```python
from build123d import *

# Parameters (mm, degrees)
F0_R     = 5
F1_DEPTH = 7
F2_DEPTH = 9
F3_R     = 5
F3_R_2   = 3
F4_DEPTH = 4
F5_DEPTH = 14
F6_R     = 1.5
F7_DEPTH = 12.5


with BuildPart() as f1:
    # F0 (on Top) → F1 (new body)
    with BuildSketch(Plane.XY):
        Circle(F0_R)
        with BuildLine():
            ThreePointArc((-2, 1.5), (0, 2.5), (2, 1.5))
            Line((2, 1.5), (3.6073317751, 1.5))
            Line((3.6073317751, 1.5), (3.6073317751, -1.5))
            Line((3.6073317751, -1.5), (2, -1.5))
            ThreePointArc((2, -1.5), (0, -2.5), (-2, -1.5))
            Line((-2, -1.5), (-3.6073317751, -1.5))
            Line((-3.6073317751, -1.5), (-3.6073317751, 1.5))
            Line((-3.6073317751, 1.5), (-2, 1.5))
        make_face(mode=Mode.SUBTRACT)
        with BuildLine():
            ThreePointArc((2, 1.5), (2.3717082451, 0.790569415), (2.5, 0))
            ThreePointArc((2.5, 0), (2.3717082451, -0.790569415), (2, -1.5))
            Line((2, -1.5), (3.6073317751, -1.5))
            Line((3.6073317751, -1.5), (3.6073317751, 1.5))
            Line((3.6073317751, 1.5), (2, 1.5))
        make_face()
        with BuildLine():
            Line((-2, 1.5), (2, 1.5))
            ThreePointArc((2, 1.5), (0, 2.5), (-2, 1.5))
        make_face()
        with BuildLine():
            ThreePointArc((-2, -1.5), (0, -2.5), (2, -1.5))
            Line((2, -1.5), (-2, -1.5))
        make_face()
        with BuildLine():
            ThreePointArc((-2, -1.5), (-2.5, 0), (-2, 1.5))
            Line((-2, 1.5), (-3.6073317751, 1.5))
            Line((-3.6073317751, 1.5), (-3.6073317751, -1.5))
            Line((-3.6073317751, -1.5), (-2, -1.5))
        make_face()
    extrude(amount=F1_DEPTH)

    # F0 (on Top) → F2 (join)
    with BuildSketch(Plane.XY):
        Circle(F0_R)
        with BuildLine():
            ThreePointArc((-2, 1.5), (0, 2.5), (2, 1.5))
            Line((2, 1.5), (3.6073317751, 1.5))
            Line((3.6073317751, 1.5), (3.6073317751, -1.5))
            Line((3.6073317751, -1.5), (2, -1.5))
            ThreePointArc((2, -1.5), (0, -2.5), (-2, -1.5))
            Line((-2, -1.5), (-3.6073317751, -1.5))
            Line((-3.6073317751, -1.5), (-3.6073317751, 1.5))
            Line((-3.6073317751, 1.5), (-2, 1.5))
        make_face(mode=Mode.SUBTRACT)
        with BuildLine():
            ThreePointArc((-2, -1.5), (-2.5, 0), (-2, 1.5))
            Line((-2, 1.5), (-3.6073317751, 1.5))
            Line((-3.6073317751, 1.5), (-3.6073317751, -1.5))
            Line((-3.6073317751, -1.5), (-2, -1.5))
        make_face()
        with BuildLine():
            ThreePointArc((2, 1.5), (2.3717082451, 0.790569415), (2.5, 0))
            ThreePointArc((2.5, 0), (2.3717082451, -0.790569415), (2, -1.5))
            Line((2, -1.5), (3.6073317751, -1.5))
            Line((3.6073317751, -1.5), (3.6073317751, 1.5))
            Line((3.6073317751, 1.5), (2, 1.5))
        make_face()
    extrude(amount=F2_DEPTH)

    # F3 (on face) → F4 (join)
    with BuildSketch(Plane(origin=(0, 0, 0), x_dir=(1, 0, 0), z_dir=(0, 0, -1))):
        Circle(F3_R)
        Circle(F3_R_2, mode=Mode.SUBTRACT)
        Circle(F3_R_2)
        with BuildLine():
            Line((2, -1.5), (-2, -1.5))
            ThreePointArc((-2, -1.5), (-2.5, 0), (-2, 1.5))
            Line((-2, 1.5), (2, 1.5))
            ThreePointArc((2, 1.5), (2.5, 0), (2, -1.5))
        make_face(mode=Mode.SUBTRACT)
        with BuildLine():
            ThreePointArc((-2, 1.5), (-2.5, 0), (-2, -1.5))
            Line((-2, -1.5), (2, -1.5))
            ThreePointArc((2, -1.5), (2.5, 0), (2, 1.5))
            Line((2, 1.5), (-2, 1.5))
        make_face()
    extrude(amount=F4_DEPTH)

    # F3 (on face) → F5 (join)
    with BuildSketch(Plane(origin=(0, 0, 0), x_dir=(1, 0, 0), z_dir=(0, 0, -1))):
        Circle(F3_R)
        Circle(F3_R_2, mode=Mode.SUBTRACT)
    extrude(amount=F5_DEPTH)

    # F6 (on Right) → F7 (cut, symmetric)
    with BuildSketch(Plane.YZ):
        with Locations((0, -5.9965602363)):
            Circle(F6_R)
    extrude(amount=F7_DEPTH, both=True, mode=Mode.SUBTRACT)


solid = f1.part
```
Geometry check sheet. Reference: the model listing, model coordinates, mm. A direction names the side the tool comes from. Give positions to 0.01 mm unless a question says otherwise; leave off trailing zeros. Order: outer loops, then holes, each group sorted by start corner. A loop starts at its lowest first (then second) coordinate and runs counter-clockwise, first axis right, second up.
1. Gauge pin test, flat ends, axial feed: pin 1 Ø1 at (x, z) = (3.5, -8.5) entering from -Y; pin 2 Ø1 at (x, y) = (-1, 2) entering from -Z; pin 3 Ø2.5 at (y, z) = (0, -6) entering from +X; pin 4 Ø1.5 at (x, y) = (0, 0.5) entering from +Z. Record the tip position at first contact, or that the pin passes through.
2. Thickness scan on L1, parallel to X at y = 0, z = -7.75; L2, parallel to Z at x = 1, y = -1.75. Record the ranges inside material, lowest first.
3. Section check C-C, the plane x = 0. Enter the section's corners in (y, z).
4. Section check B-B, the plane z = -6.25. Enter the section's corners in (x, y).
5. Section check A-A, the plane y = 0. Enter the section's corners in (x, z).
6. Access from +Z, -Z, +X, -X, +Y, -Y to the whole of each face (thin tool, end or side, straight path). Record for faces 1 (the face through (0, 1.5, 3)), 2 (the face through (2, -2, 9)).
7. Release check for a two-part mould opening along Y. For faces 3 (the face through (0, 0, -4)), 4 (the face through (-3, 0, -9)), 5 (the face through (-0.1, 3.3, -14)), 6 (the face through (4.77, -1.5, -2.34)) record: pulls with the +Y half, pulls with the -Y half, needs draft (parallel to the pull), parting line crosses it, or undercut.
8. Section check D-D, the plane x = -3.75. Enter the section's corners in (y, z).
Values follow:
1. pin 1: stops at y = -4
1. pin 2: stops at z = -4
1. pin 3: passes through
1. pin 4: stops at z = 0
2. L1: x = -5 to -3, 3 to 5
2. L2: z = -4 to 7
3. outline: (-5, -14) - (-3, -14) - (-3, -4) - (3, -4) - (3, -14) - (5, -14) - (5, 9) - (2.5, 9) - (2.5, 7) - (1.5, 7) - (1.5, 0) - (-1.5, 0) - (-1.5, 7) - (-2.5, 7) - (-2.5, 9) - (-5, 9) - close
4. outline: (-4.78, -1.48) arc R5 ccw to (4.78, -1.48) - (2.61, -1.48) arc R3 cw to (-2.61, -1.48) - close; (-4.78, 1.48) - (-2.61, 1.48) arc R3 cw to (2.61, 1.48) - (4.78, 1.48) arc R5 ccw to start
5. outline: (-5, -14) - (-3, -14) - (-3, -7.5) - (-5, -7.5) - close; (-5, -4.5) - (-3, -4.5) - (-3, -4) - (3, -4) - (3, -4.5) - (5, -4.5) - (5, 9) - (2.5, 9) - (2.5, 0) - (-2.5, 0) - (-2.5, 9) - (-5, 9) - close; (3, -14) - (5, -14) - (5, -7.5) - (3, -7.5) - close
6. face 1: +Z
6. face 2: +Z, +X, -X, +Y, -Y
7. face 3: undercut
7. face 4: undercut
7. face 5: needs draft
7. face 6: parting line crosses it
8. outline: (-3.31, -14) - (3.31, -14) - (3.31, 9) - (-3.31, 9) - close; hole circle Ø3 at (0, -6)
